Geometry check sheet. Reference: the model listing, model coordinates, mm. Round coordinates to 2 decimals unless told otherwise and drop trailing zeros. Write each loop counter-clockwise with the first axis right and the second up, starting at its lowest first coordinate (ties: lowest second). Pieces come first, ordered by that corner, then holes. Notation, with made-up numbers: M 49,65 L 64,65 A9 ccw 64,71 Z; hole C 84.25,43.25 d8. An arc over 180 degrees is marked long. Put each result on its own line as item: value. Start each with the question number.
(1) Section check A-A on z = 1. Record the cut outline in (x, y), then the cut area to 3 significant figures.
(2) Gauge pin test, flat ends, axial feed: pin 1 (1.5 mm diameter, centred on x = -14, z = 0.5, fed in from -Y); pin 2 (4 mm diameter, centred on x = 10, y = 1, fed in from -Z); pin 3 (4 mm diameter, centred on x = 0, y = 11, fed in from -Z); pin 4 (8 mm diameter, centred on x = 0, y = -1.5, fed in from +Z). Record the tip position at first contact, or that the pin passes through.
(3) Material ranges on probe 1 along Y at (x, z) = (0, 1); probe 2 along Y at (x, z) = (0, 2.5); probe 3 along X at (y, z) = (-2, 0.75), recorded low to high.
(4) Section check B-B on x = 0. Count the separate pieces of the cut face and the enclosed holes in it, then the cut area to 3 significant figures.
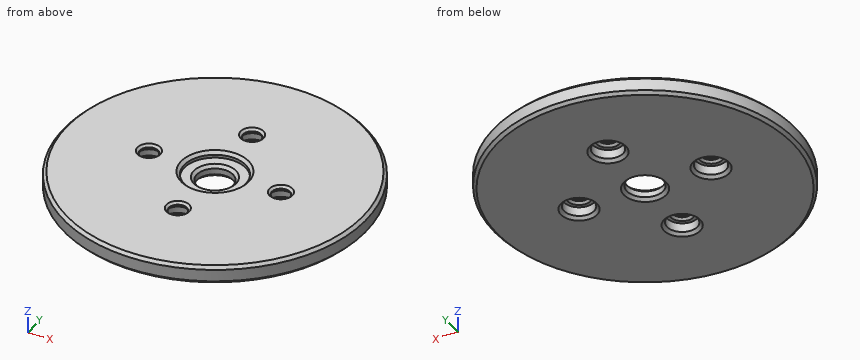
from build123d import *

# Parameters (mm, degrees)
SKETCH_R        = 25
SKETCH_R_2      = 1.5
PAD_DEPTH       = 3
SKETCH002_R     = 3
POCKET_DEPTH    = 4
SKETCH001_R     = 5.1
POCKET001_DEPTH = 1
SKETCH003_R     = 2.5
POCKET002_DEPTH = 2
CHAMFER_SIZE    = 0.5
CHAMFER001_SIZE = 0.5
CHAMFER002_SIZE = 0.5
CHAMFER003_SIZE = 0.4
CHAMFER004_SIZE = 0.5


with BuildPart() as part:
    # Sketch → Pad (new body)
    with BuildSketch(Plane.XY):
        Circle(SKETCH_R)
        with Locations((0, 11)):
            Circle(SKETCH_R_2, mode=Mode.SUBTRACT)
        with Locations((-11, 0)):
            Circle(SKETCH_R_2, mode=Mode.SUBTRACT)
        with Locations((0, -11)):
            Circle(SKETCH_R_2, mode=Mode.SUBTRACT)
        with Locations((11, 0)):
            Circle(SKETCH_R_2, mode=Mode.SUBTRACT)
    extrude(amount=PAD_DEPTH)

    # Sketch002 (on Face7 of Pad) → Pocket (cut)
    with BuildSketch(Plane.XY.offset(3)):
        Circle(SKETCH002_R)
    extrude(amount=-POCKET_DEPTH, mode=Mode.SUBTRACT)

    # Sketch001 (on Face7 of Pad) → Pocket001 (cut)
    with BuildSketch(Plane.XY.offset(3)):
        Circle(SKETCH001_R)
    extrude(amount=-POCKET001_DEPTH, mode=Mode.SUBTRACT)

    # Sketch003 (on Face2 of Pocket001) → Pocket002 (cut)
    with BuildSketch(Plane(origin=(0, 0, 0), x_dir=(1, 0, 0), z_dir=(0, 0, -1))):
        with Locations((0, 11)):
            Circle(SKETCH003_R)
        with Locations((11, 0)):
            Circle(SKETCH003_R)
        with Locations((0, -11)):
            Circle(SKETCH003_R)
        with Locations((-11, 0)):
            Circle(SKETCH003_R)
    extrude(amount=-POCKET002_DEPTH, mode=Mode.SUBTRACT)

    # Chamfer
    chamfer_edges = [part.edges().sort_by_distance(p)[0] for p in [
        (-25, 0, 3),
        (-25, 0, 0),
    ]]
    chamfer(chamfer_edges, length=CHAMFER_SIZE)

    # Chamfer001
    chamfer001_edges = [part.edges().sort_by_distance(p)[0] for p in [
        (-5.1, 0, 3),
    ]]
    chamfer(chamfer001_edges, length=CHAMFER001_SIZE)

    # Chamfer002
    chamfer002_edges = [part.edges().sort_by_distance(p)[0] for p in [
        (-3, 0, 2),
        (-3, 0, 0),
    ]]
    chamfer(chamfer002_edges, length=CHAMFER002_SIZE)

    # Chamfer003
    chamfer003_edges = [part.edges().sort_by_distance(p)[0] for p in [
        (-1.5, 11, 3),
        (-1.5, 11, 2),
        (-12.5, 0, 3),
        (-12.5, 0, 2),
        (9.5, 0, 3),
        (9.5, 0, 2),
        (-1.5, -11, 3),
        (-1.5, -11, 2),
    ]]
    chamfer(chamfer003_edges, length=CHAMFER003_SIZE)

    # Chamfer004
    chamfer004_edges = [part.edges().sort_by_distance(p)[0] for p in [
        (-13.5, 0, 0),
        (-2.5, 11, 0),
        (8.5, 0, 0),
        (-2.5, -11, 0),
    ]]
    chamfer(chamfer004_edges, length=CHAMFER004_SIZE)


solid = part.part
Answers follow:
1. outline: C 0,0 d50; hole C -11,0 d5; hole C 0,0 d6; hole C 0,-11 d5; hole C 0,11 d5; hole C 11,0 d5
1. area: 1,860 mm^2
2. pin 1: stops at y = -21.2
2. pin 2: stops at z = 0
2. pin 3: stops at z = 2
2. pin 4: stops at z = 2.9
3. probe 1: y = -25 to -13.5, -8.5 to -3, 3 to 8.5, 13.5 to 25
3. probe 2: y = -25 to -12.5, -9.5 to -5.1, 5.1 to 9.5, 12.5 to 25
3. probe 3: x = -24.92 to -12.5, -9.5 to -2.24, 2.24 to 9.5, 12.5 to 24.92
4. separate pieces: 4
4. enclosed holes: 0
4. area: 99.4 mm^2
